Print and shaded views of the part. All mm, measured from the part's lowest x, y and z. Give positions to 0.01 mm unless a question says otherwise; leave off trailing zeros. Write each loop counter-clockwise with the first axis right and the second up, starting at its lowest first coordinate (ties: lowest second). Pieces come first, ordered by that corner, then holes.
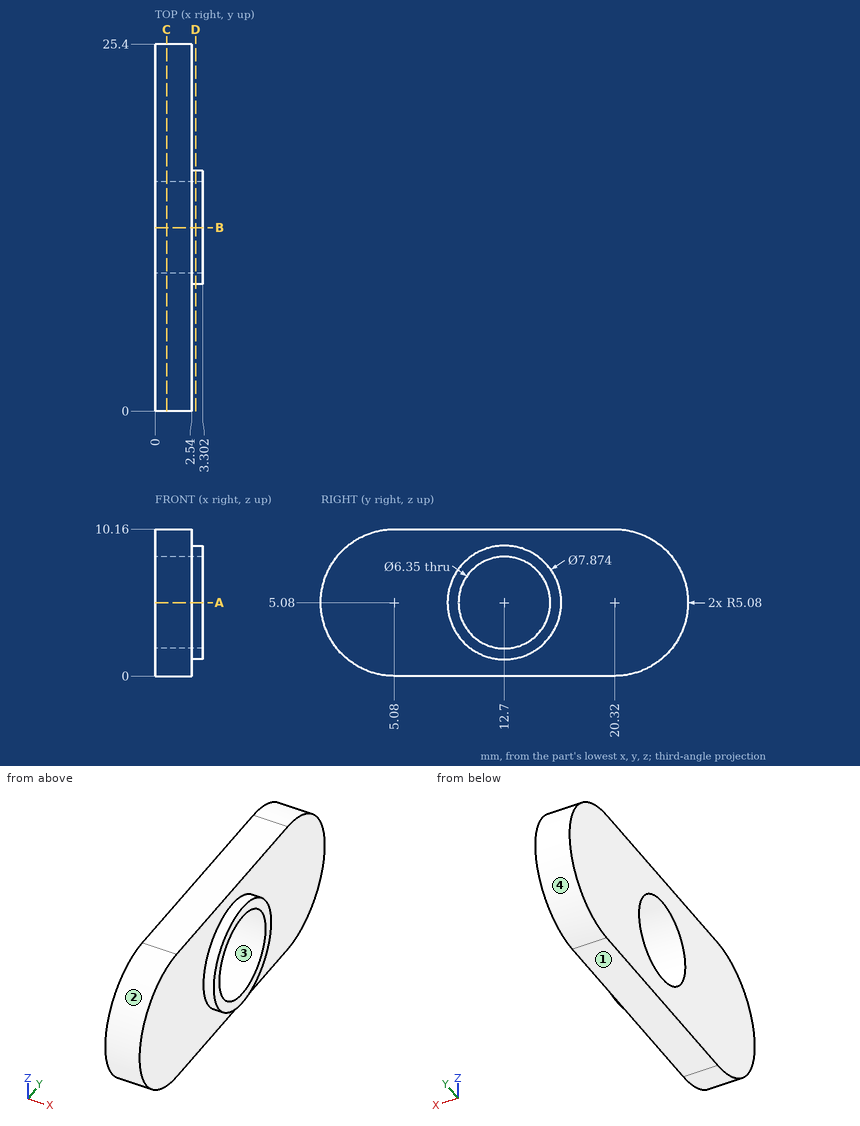
1. Saw through at D-D on x = 2.8. Give the cut face in (y, z) (3 decimals).
2. Drill centre lines: line 1 along Y through (x, z) = (1.9, 5.08) (3 decimals); line 2 along Y through (x, z) = (2.65, 5.08) (3 decimals); line 3 along X through (y, z) = (18.5, 4.5). Where is each one in solid material? Low to high.
3. Saw through at A-A on z = 5.08. Give the cut face in (x, y) (3 decimals).
4. Saw through at C-C on x = 0.8. Give the cut face in (y, z) (3 decimals).
5. Saw through at B-B on y = 12.7. Give the cut face in (x, z) (3 decimals).
6. Mould opens along Y. For the marked faces 1, 2, 3 and 4 say: pulls with the +Y half, pulls with the -Y half, needs draft (parallel to the pull), parting line crosses it, or undercut.
Outcome:
1. outline: circle Ø7.874 at (12.7, 5.08); hole circle Ø6.35 at (12.7, 5.08)
2. line 1: y = 0 to 9.525, 15.875 to 25.4
2. line 2: y = 8.763 to 9.525, 15.875 to 16.637
2. line 3: x = 0 to 2.54
3. outline: (0, 0) - (2.54, 0) - (2.54, 8.763) - (3.302, 8.763) - (3.302, 9.525) - (0, 9.525) - close; (0, 15.875) - (3.302, 15.875) - (3.302, 16.637) - (2.54, 16.637) - (2.54, 25.4) - (0, 25.4) - close
4. outline: (5.08, 0) - (20.32, 0) arc R5.08 ccw to (20.32, 10.16) - (5.08, 10.16) arc R5.08 ccw to start; hole circle Ø6.35 at (12.7, 5.08)
5. outline: (0, 0) - (2.54, 0) - (2.54, 1.143) - (3.302, 1.143) - (3.302, 1.905) - (0, 1.905) - close; (0, 8.255) - (3.302, 8.255) - (3.302, 9.017) - (2.54, 9.017) - (2.54, 10.16) - (0, 10.16) - close
6. face 1: needs draft
6. face 2: pulls with the -Y half
6. face 3: undercut
6. face 4: pulls with the +Y half
